Build history of the part. All positions in model axes, mm. Face numbers are marked on the shaded views. Coordinates: 2 decimals unless noted, no trailing zeros. Order: outer loops, then holes, each group sorted by start corner. A loop starts at its lowest first (then second) coordinate and runs counter-clockwise, first axis right, second up. Notation, with made-up numbers: M -5.5,47.25 L 9.5,47.25 A26 ccw 9.5,85.25 Z; hole C 49,71 d3. An arc over 180 degrees is marked long. Use a Markdown table: item, result. Add a question column.
from build123d import *

# Parameters (mm, degrees)
SKETCH1_R                               = 15
BOSS_EXTRUDE1_DEPTH                     = 27
CBORE_FOR_M6_HEX_HEAD_BOLT1_D           = 20
CBORE_FOR_M6_HEX_HEAD_BOLT1_CBORE_D     = 22
CBORE_FOR_M6_HEX_HEAD_BOLT1_CBORE_DEPTH = 12
BOSS_EXTRUDE2_START                     = 1
SKETCH5_R                               = 15
BOSS_EXTRUDE2_DEPTH                     = 1
CUT_EXTRUDE1_DEPTH                      = 35.336569427
CUT_EXTRUDE1_DEPTH_BACK                 = 35.336569427
SKETCH4_R                               = 2.5


with BuildPart() as part:
    # Sketch1 → Boss-Extrude1 (new body)
    with BuildSketch(Plane.XY):
        Circle(SKETCH1_R)
    extrude(amount=BOSS_EXTRUDE1_DEPTH)

    # CBORE for M6 Hex Head Bolt1 (through all)
    with Locations(Plane.XY.offset(27)):
        with Locations((0, 0)):
            CounterBoreHole(CBORE_FOR_M6_HEX_HEAD_BOLT1_D / 2, CBORE_FOR_M6_HEX_HEAD_BOLT1_CBORE_D / 2, CBORE_FOR_M6_HEX_HEAD_BOLT1_CBORE_DEPTH)

    # Sketch5 → Boss-Extrude2 (add)
    with BuildSketch(Plane(origin=(0, 0, 0), x_dir=(-1, 0, 0), z_dir=(0, 0, -1)).offset(BOSS_EXTRUDE2_START)):
        Circle(SKETCH5_R)
    extrude(amount=-BOSS_EXTRUDE2_DEPTH)

    # Sketch4 → Cut-Extrude1 (cut, two sides: drawn at the far end of the back side and taken through both)
    with BuildSketch(Plane(origin=(0, 0, 0), x_dir=(1, 0, 0), z_dir=(0, 1, 0)).offset(-CUT_EXTRUDE1_DEPTH_BACK)):
        with Locations(Location((0, -12, 0), (0, 0, 270))):
            Circle(SKETCH4_R)
    extrude(amount=CUT_EXTRUDE1_DEPTH + CUT_EXTRUDE1_DEPTH_BACK, mode=Mode.SUBTRACT)


solid = part.part
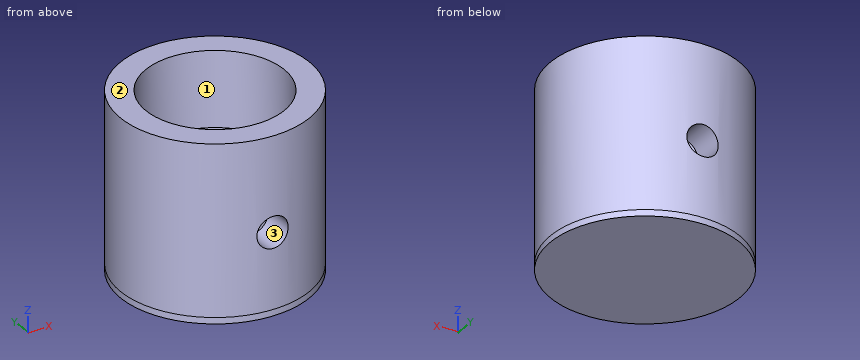
(1) Drop flat-ended pins along their axis: P1, Ø10, axis at x = 4, y = -2, coming from the +Z side; P2, Ø10, axis at y = -3, z = 15, coming from the +X side; P3, Ø2, axis at y = -9, z = 8, coming from the +X side; P4, Ø8, axis at x = 7, z = 16, coming from the -Y side. Give the stop position or say it passes through.
(2) Slice it at D-D on y = -4. Give the cut face in (x, z), and give its area (3 significant figures).
(3) Slice it at C-C on y = 12.5. Give the cut face in (x, z), and give its area (3 significant figures).
(4) Slice it at B-B on z = 12. Give the cut face in (x, y).
(5) Mould opens along X. For the marked faces 1, 2 and 3 say: released by +X, released by -X, zero draft, split by the parting line, or undercut.
(6) Drill centre lines: line 1 along Y through (x, z) = (0, 8); line 2 along Y through (x, z) = (0, 21); line 3 along Z through (x, y) = (6, 9). Where is each one in solid material? Low to high. Write a range as from..to.
(7) Slice it at A-A on x = 0. Give the cut face in (y, z).
Solutions:
| question | item | result |
|---|---|---|
| 1 | P1 | z = 0 |
| 1 | P2 | x = 15 |
| 1 | P3 | x = 12.69 |
| 1 | P4 | y = -14.7 |
| 2 | outline | M -14.46,-1 L 14.46,-1 L 14.46,27 L 10.25,27 L 10.25,15 L 9.17,15 L 9.17,0 L -9.17,0 L -9.17,15 L -10.25,15 L -10.25,27 L -14.46,27 Z |
| 2 | area | 289 mm² |
| 3 | outline | M -8.29,-1 L 8.29,-1 L 8.29,27 L -8.29,27 Z; hole C 0,12 d5 |
| 3 | area | 445 mm² |
| 4 | outline | M -2.5,-14.79 L -2.5,-9.68 A10 cw -2.5,9.68 L -2.5,14.79 A15 ccw Z; M 2.5,-14.79 A15 ccw 2.5,14.79 L 2.5,9.68 A10 cw 2.5,-9.68 Z |
| 5 | face 1 | undercut |
| 5 | face 2 | zero draft |
| 5 | face 3 | undercut |
| 6 | line 1 | -15..-10, 10..15 |
| 6 | line 2 | -15..-11, 11..15 |
| 6 | line 3 | -1..15 |
| 7 | outline | M -15,-1 L 15,-1 L 15,9.5 L 10,9.5 L 10,0 L -10,0 L -10,9.5 L -15,9.5 Z; M -15,14.5 L -10,14.5 L -10,15 L -11,15 L -11,27 L -15,27 Z; M 10,14.5 L 15,14.5 L 15,27 L 11,27 L 11,15 L 10,15 Z |
